```python
from build123d import *

# Parameters (mm, degrees)
F0_W      = 25
F0_H      = 25
F1_DEPTH  = 3.6
F3_DEPTH  = 0.6
F4_W      = 4.6
F4_H      = 2.6
F5_DEPTH  = 0.9
F6_R      = 1.6
F7_DEPTH  = 1.2
F8_R      = 0.2
F9_R      = 0.8
F10_DEPTH = 8


with BuildPart() as f1:
    # F0 (on Top) → F1 (new body)
    with BuildSketch(Plane.XY):
        Rectangle(F0_W, F0_H)
    extrude(amount=F1_DEPTH)

    # F2 (on face) → F3 (cut)
    with BuildSketch(Plane.XY.offset(3.6)):
        Polygon((-2.968572, 9.5), (-8.568572, 9.5), (-8.568572, 4.4), (-7.368572, 4.4), (-7.368572, 0.2), (-4.168572, 0.2), (-4.168572, 4.4), (-2.968572, 4.4), align=None)
        Polygon((7.511108, 4.5), (1.911108, 4.5), (1.911108, -0.7), (3.261108, -0.7), (3.261108, -4.8), (6.161108, -4.8), (6.161108, -0.7), (7.511108, -0.7), align=None)
    extrude(amount=-F3_DEPTH, mode=Mode.SUBTRACT)

    # F4 (on face) → F5 (cut)
    with BuildSketch(Plane.XY.offset(3.6)):
        Polygon((-7.552263, -2.098206), (-9.040832, 2.254283), (-11.500935, 1.412918), (-10.012366, -2.939571), align=None)
        Polygon((-0.058017, 1.566966), (-2.565525, 2.254283), (-3.781548, -2.182077), (-1.27404, -2.869394), align=None)
        Polygon((0.855684, -3.437364), (-1.366318, -4.78744), (1.02228, -8.718675), (3.244282, -7.368598), align=None)
        Polygon((10.624292, -3.622611), (8.143836, -2.843295), (6.765044, -7.231795), (9.245501, -8.011112), align=None)
        with Locations((-5.702388, -5.56096)):
            Rectangle(F4_W, F4_H)
    extrude(amount=-F5_DEPTH, mode=Mode.SUBTRACT)

    # F6 (on face) → F7 (cut)
    with BuildSketch(Plane(origin=(0, 0, 0), x_dir=(1, 0, 0), z_dir=(0, 0, -1))):
        with Locations((0, 7.5)):
            Circle(F6_R)
        Circle(F6_R)
        with Locations((0, -7.5)):
            Circle(F6_R)
        with Locations((-7.5, 0)):
            Circle(F6_R)
        with Locations((7.5, 0)):
            Circle(F6_R)
    extrude(amount=-F7_DEPTH, mode=Mode.SUBTRACT)

    # F8
    f8_edges = [f1.edges().sort_by_distance(p)[0] for p in [
        (-12.5, -12.5, 1.8),
        (12.5, -12.5, 1.8),
        (12.5, 12.5, 1.8),
        (-12.5, 12.5, 1.8),
    ]]
    fillet(f8_edges, radius=F8_R)

    # F9 (on face) → F10 (cut)
    with BuildSketch(Plane.XZ.offset(12.5)):
        with Locations((-10, 1.4)):
            Circle(F9_R)
        with Locations((10, 1.4)):
            Circle(F9_R)
    extrude(amount=-F10_DEPTH, mode=Mode.SUBTRACT)


solid = f1.part
```
Work out the finished part from the listing and answer in its coordinate system (mm). A direction names the side the tool comes from. Give positions to 0.01 mm unless a question says otherwise; leave off trailing zeros. Order: outer loops, then holes, each group sorted by start corner. A loop starts at its lowest first (then second) coordinate and runs counter-clockwise, first axis right, second up. Notation, with made-up numbers: (-2.75, 66) - (43.25, 66) arc R26 ccw to (43.25, 93) - close; hole circle Ø6 at (32.25, 33). An arc over 180 degrees is marked (long way). One line per item, written item: value. Start each with the question number.
1. For a pull along Y with two mould halves and no side action, classify faces 1 (the face through (0, -12.5, 2)), 2 (the face through (0, 12.5, 2)), 3 (the face through (0, 3, 0)), 4 (the face through (-2.55, -2.52, 3.16)) as released by +Y, released by -Y, zero draft, split by the parting line, or undercut.
2. Consider line 1 (X direction, y = 7.5, z = 0.3); line 2 (Z direction, x = 10, y = -10.75). Determine where each line is inside the solid, lowest interval first.
3. Section A-A, the plane y = 7.5 is taken. Write down the section's boundary in (x, z).
4. Section C-C, the plane z = 3.3 is taken. Count the separate pieces of the cut face and the enclosed holes in it, then the cut area to 3 significant figures.
5. Which of the six approach directions +Z, -Z, +X, -X, +Y, -Y give full straight-line access (tool end or side, diameter ignored) to faces 5 (the face through (7, 0, 1.2)), 6 (the face through (-10, -4.5, 1)), 7 (the face through (-12.5, 0, 2)), 8 (the face through (9, -5, 2.7))?
6. This flat-tipped pin is pushed along its axis until it touches: pin 1 Ø1.6 at (x, y) = (-0.5, 8) entering from -Z. Where does it stop, or does it pass through?
7. Section B-B, the plane x = -4.5 is taken. Write down the section's boundary in (y, z).
Filled sheet:
1. face 1: released by -Y
1. face 2: released by +Y
1. face 3: zero draft
1. face 4: undercut
2. line 1: -12.5 to -1.6, 1.6 to 12.5
2. line 2: 0 to 0.6, 2.2 to 3.6
3. outline: (-12.5, 0) - (-1.6, 0) - (-1.6, 1.2) - (1.6, 1.2) - (1.6, 0) - (12.5, 0) - (12.5, 3.6) - (-2.97, 3.6) - (-2.97, 3) - (-8.57, 3) - (-8.57, 3.6) - (-12.5, 3.6) - close
4. separate pieces: 1
4. enclosed holes: 7
4. area: 482 mm²
5. face 5: -Z
5. face 6: -Y
5. face 7: +Z, -Z, -X, +Y, -Y
5. face 8: +Z
6. pin 1: z = 1.2
7. outline: (-12.5, 0) - (12.5, 0) - (12.5, 3.6) - (9.5, 3.6) - (9.5, 3) - (0.2, 3) - (0.2, 3.6) - (-4.26, 3.6) - (-4.26, 2.7) - (-6.86, 2.7) - (-6.86, 3.6) - (-12.5, 3.6) - close
